Here's how the part is built. I have some questions about the finished solid (model axes, mm). Round coordinates to 2 decimals unless told otherwise and drop trailing zeros. Order: outer loops, then holes, each group sorted by start corner. A loop starts at its lowest first (then second) coordinate and runs counter-clockwise, first axis right, second up. Notation, with made-up numbers: (-37, -21) - (-11, -21) arc R22 ccw to (-11, 3) - close; hole circle Ø1 at (62, -21.5). An arc over 180 degrees is marked (long way). One line per item, written item: value.
from build123d import *

# Parameters (mm, degrees)
SKETCH1_R           = 3
BOSS_EXTRUDE2_DEPTH = 3
SKETCH4_R           = 9.5
CUT_EXTRUDE2_DEPTH  = 10
SKETCH5_R           = 2
CUT_EXTRUDE3_DEPTH  = 3
SKETCH6_R           = 2.25
CUT_EXTRUDE4_DEPTH  = 3
SKETCH7_R           = 2.25
CUT_EXTRUDE5_DEPTH  = 10


with BuildPart() as part:
    # Sketch1 → Boss-Extrude2 (new body)
    with BuildSketch(Plane.XY):
        with BuildLine():
            Line((-34.17966517, 1.656542757), (-34.17966517, 41.656542757))
            Line((-34.17966517, 41.656542757), (-64.17966517, 41.656542757))
            Line((-64.17966517, 41.656542757), (-64.17966517, -118.343457243))
            ThreePointArc((-64.17966517, -118.343457243), (0.82033483, -133.158398897), (65.82033483, -118.343457243))
            Line((65.82033483, -118.343457243), (65.82033483, 41.656542757))
            Line((65.82033483, 41.656542757), (35.82033483, 41.656542757))
            Line((35.82033483, 41.656542757), (35.82033483, 1.656542757))
            ThreePointArc((35.82033483, 1.656542757), (0.82033483, -7.721678978), (-34.17966517, 1.656542757))
        make_face()
        with Locations((60.82033483, 20.554474708)):
            Circle(SKETCH1_R, mode=Mode.SUBTRACT)
        with Locations((42.82033483, 20.554474708)):
            Circle(SKETCH1_R, mode=Mode.SUBTRACT)
        with Locations(Location((-59.17966517, 20.554474708, 0), (0, 0, 180))):
            Circle(SKETCH1_R, mode=Mode.SUBTRACT)
        with Locations(Location((-41.17966517, 20.554474708, 0), (0, 0, 180))):
            Circle(SKETCH1_R, mode=Mode.SUBTRACT)
    extrude(amount=BOSS_EXTRUDE2_DEPTH)

    # Sketch4 → Cut-Extrude2 (cut)
    with BuildSketch(Plane.XY.offset(3)):
        with Locations((0.82033483, -110.721678978)):
            Circle(SKETCH4_R)
    extrude(amount=-CUT_EXTRUDE2_DEPTH, mode=Mode.SUBTRACT)

    # Sketch5 → Cut-Extrude3 (cut)
    with BuildSketch(Plane(origin=(0, 0, 0), x_dir=(-1, 0, 0), z_dir=(0, 0, -1))):
        with Locations((-14.82033483, -121.721678978)):
            Circle(SKETCH5_R)
        with Locations((-14.82033483, -81.721678978)):
            Circle(SKETCH5_R)
        with Locations((13.17966517, -81.721678978)):
            Circle(SKETCH5_R)
        with Locations((13.17966517, -121.721678978)):
            Circle(SKETCH5_R)
    extrude(amount=-CUT_EXTRUDE3_DEPTH, mode=Mode.SUBTRACT)

    # Sketch6 → Cut-Extrude4 (cut)
    with BuildSketch(Plane(origin=(0, 0, 0), x_dir=(-1, 0, 0), z_dir=(0, 0, -1))):
        with Locations((-26.170124502, -42.870278614)):
            Circle(SKETCH6_R)
        with Locations((-26.339734066, -15.290278614)):
            Circle(SKETCH6_R)
        with Locations((24.529454842, -15.290278614)):
            Circle(SKETCH6_R)
        with Locations((24.699064406, -42.870278614)):
            Circle(SKETCH6_R)
    extrude(amount=-CUT_EXTRUDE4_DEPTH, mode=Mode.SUBTRACT)

    # Sketch7 → Cut-Extrude5 (cut)
    with BuildSketch(Plane.XY.offset(3)):
        with Locations((-58.050753667, -112.076170868)):
            Circle(SKETCH7_R)
        with Locations((-58.050753667, -94.961890213)):
            Circle(SKETCH7_R)
        with Locations((-58.050753667, -76.250276697)):
            Circle(SKETCH7_R)
        with Locations((-58.050753667, -55.028568685)):
            Circle(SKETCH7_R)
        with Locations((-58.735324893, -10.759629391)):
            Circle(SKETCH7_R)
        with Locations((-58.735324893, 31.901332055)):
            Circle(SKETCH7_R)
        with Locations((59.892687825, -112.115366711)):
            Circle(SKETCH7_R)
        with Locations((59.892687825, -90.405584769)):
            Circle(SKETCH7_R)
        with Locations((59.892687825, -70.121992882)):
            Circle(SKETCH7_R)
        with Locations((59.892687825, -50.255835401)):
            Circle(SKETCH7_R)
        with Locations((59.892687825, -8.825910752)):
            Circle(SKETCH7_R)
        with Locations((59.892687825, 33.03311017)):
            Circle(SKETCH7_R)
    extrude(amount=-CUT_EXTRUDE5_DEPTH, mode=Mode.SUBTRACT)


solid = part.part
Q1. If we section it at A-A, the plane y = 3.5: Please give me the cut outline in (x, z).
Results list:
outline: (-64.18, 0) - (-34.18, 0) - (-34.18, 3) - (-64.18, 3) - close; (35.82, 0) - (65.82, 0) - (65.82, 3) - (35.82, 3) - close
Q2. If we section it at D-D, the plane x = -4.5: Please give me the cut outline in (y, z), then the cut area to 3 significant figures.
Results list:
outline: (-133.06, 0) - (-118.59, 0) - (-118.59, 3) - (-133.06, 3) - close; (-102.85, 0) - (-7.52, 0) - (-7.52, 3) - (-102.85, 3) - close
area: 329 mm²
Q3. If I drill on line 1 along X through (y, z) = (-15.5, 0.55); line 2 along Y through (x, z) = (-14, 1.8); line 3 along X through (y, z) = (27, 2.95), over which ranges is the centre line in solid material (lowest first)?
Results list:
line 1: -64.18 to -26.77, -22.29 to 24.1, 28.58 to 65.82
line 2: -132.42 to -123.55, -119.9 to -83.55, -79.9 to -6.13
line 3: -64.18 to -34.18, 35.82 to 65.82
Q4. If we section it at C-C, the plane z = 2.1: Give the number of separate pieces and of enclosed holes in the cut face, then the cut area to 3 significant figures.
Results list:
separate pieces: 1
enclosed holes: 25
area: 18,200 mm²
Q5. We'd pull the mould along Y, two halves only. Please class faces 1 (the cylindrical face through (-22.28, -15.19, 1.48)), 2 (the flat face through (0, -45, 3)): released by +Y, released by -Y, zero draft, split by the parting line, or undercut.
Results list:
face 1: undercut
face 2: zero draft
Q6. If we section it at B-B, the plane x = 26: Please give me the cut outline in (y, z), then the cut area to 3 significant figures.
Results list:
outline: (-131.03, 0) - (-45.11, 0) - (-45.11, 3) - (-131.03, 3) - close; (-40.63, 0) - (-17.51, 0) - (-17.51, 3) - (-40.63, 3) - close; (-13.07, 0) - (-3.04, 0) - (-3.04, 3) - (-13.07, 3) - close
area: 357 mm²
